Here's how the part is built. I have some questions about the finished solid (model axes, mm). Face numbers are marked on the shaded views. Round coordinates to 2 decimals unless told otherwise and drop trailing zeros. Write each loop counter-clockwise with the first axis right and the second up, starting at its lowest first coordinate (ties: lowest second). Pieces come first, ordered by that corner, then holes. Notation, with made-up numbers: M 43.25,-18.5 L 99.25,-18.5 A19 cw 99.25,-1.5 Z; hole C -33,-20.5 d7. An arc over 180 degrees is marked long. Write item = value, one per line. Start each with the question number.
(1) If we mould it in two halves opening along X, with no side actions, what happens to the marked faces 1, 2 and 3? For each: released by +X, released by -X, zero draft, split by the parting line, or undercut.
(2) I want a section at B-B (z = 11). List the corners of the cut face in (x, y) for me, and give its area (3 significant figures).
(3) I want a section at D-D (y = 17.75). List the corners of the cut face in (x, z) for me, and give its area (3 significant figures).
(4) Will these pins go through, and if not, where does the flat tip stop? pin 1 Ø8 at (y, z) = (4.5, 19) entering from +X; pin 2 Ø10 at (y, z) = (11, -2) entering from -X; pin 3 Ø1 at (y, z) = (9.5, 18.5) entering from -X.
(5) I want a section at C-C (y = 5). List the corners of the cut face in (x, z) for me.
(6) I want a section at A-A (x = -25.5). List the corners of the cut face in (y, z) for me.
(7) I need wall thicknesses on line 1 along X through (y, z) = (21.4, 0); line 2 along X through (y, z) = (20.5, 11); line 3 along Y through (x, z) = (-20, -2.5). Which ranges of each line are inside material? Lowest first, please.
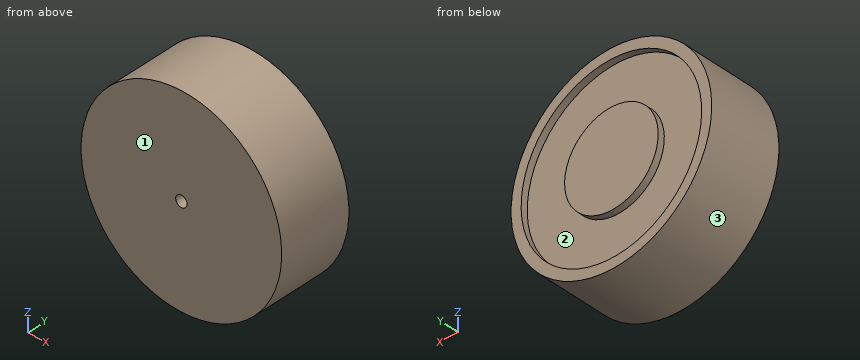
```python
from build123d import *

# Parameters (mm, degrees)
SKETCH1_R                = 30
BOSS_EXTRUDE1_DEPTH      = 22
SKETCH2_R                = 27
CUT_EXTRUDE1_DEPTH       = 2
SKETCH3_R                = 14
BOSS_EXTRUDE2_DEPTH      = 2
M3_CLEARANCE_HOLE1_D     = 3.4
M3_CLEARANCE_HOLE1_DEPTH = 7
M3_CLEARANCE_HOLE1_TIP   = 1.021463052


with BuildPart() as part:
    # Sketch1 → Boss-Extrude1 (new body)
    with BuildSketch(Plane(origin=(0, 0, 0), x_dir=(1, 0, 0), z_dir=(0, 1, 0))):
        with Locations(Location((0, 0, 0), (0, 0, 270))):
            Circle(SKETCH1_R)
    extrude(amount=BOSS_EXTRUDE1_DEPTH)

    # Sketch2 → Cut-Extrude1 (cut)
    with BuildSketch(Plane(origin=(0, 22, 0), x_dir=(1, 0, 0), z_dir=(0, 1, 0))):
        with Locations(Location((0, 0, 0), (0, 0, 270))):
            Circle(SKETCH2_R)
    extrude(amount=-CUT_EXTRUDE1_DEPTH, mode=Mode.SUBTRACT)

    # Sketch3 → Boss-Extrude2 (add)
    with BuildSketch(Plane(origin=(0, 20, 0), x_dir=(1, 0, 0), z_dir=(0, 1, 0))):
        with Locations(Location((0, 0, 0), (0, 0, 270))):
            Circle(SKETCH3_R)
    extrude(amount=BOSS_EXTRUDE2_DEPTH)

    # M3 Clearance Hole1
    with Locations(Plane(origin=(0, 0, 0), x_dir=(-1, 0, 0), z_dir=(0, -1, 0))):
        with Locations((0, 0)):
            Hole(M3_CLEARANCE_HOLE1_D / 2, depth=M3_CLEARANCE_HOLE1_DEPTH)
            with Locations((0, 0, -(M3_CLEARANCE_HOLE1_DEPTH + M3_CLEARANCE_HOLE1_TIP / 2))):  # 118° drill point
                Cone(0, M3_CLEARANCE_HOLE1_D / 2, M3_CLEARANCE_HOLE1_TIP, mode=Mode.SUBTRACT)


solid = part.part
```
Returned:
q1.face_1 = zero draft
q1.face_2 = undercut
q1.face_3 = split by the parting line
q2.outline = M -27.91,0 L 27.91,0 L 27.91,22 L 24.66,22 L 24.66,20 L 8.66,20 L 8.66,22 L -8.66,22 L -8.66,20 L -24.66,20 L -24.66,22 L -27.91,22 Z
q2.area = 1,160 mm²
q3.outline = C 0,0 d60
q3.area = 2,830 mm²
q4.pin_1 = 25.98
q4.pin_2 = -30
q4.pin_3 = -24
q5.outline = C 0,0 d60; hole C 0,0 d3.4
q6.outline = M 0,-15.8 L 22,-15.8 L 22,-8.87 L 20,-8.87 L 20,8.87 L 22,8.87 L 22,15.8 L 0,15.8 Z
q7.line_1 = -30 to -27, -14 to 14, 27 to 30
q7.line_2 = -27.91 to -24.66, -8.66 to 8.66, 24.66 to 27.91
q7.line_3 = 0 to 20
